from build123d import *

# Parameters (mm, degrees)
SKETCH1_W           = 35
SKETCH1_H           = 18
BOSS_EXTRUDE1_DEPTH = 2
SKETCH2_W           = 5
SKETCH2_H           = 6
BOSS_EXTRUDE2_DEPTH = 1.2
SKETCH3_W           = 5
SKETCH3_H           = 1
BOSS_EXTRUDE3_DEPTH = 1


with BuildPart() as part:
    # Sketch1 → Boss-Extrude1 (new body)
    with BuildSketch(Plane(origin=(0, 0, 0), x_dir=(1, 0, 0), z_dir=(0, 1, 0))):
        Rectangle(SKETCH1_W, SKETCH1_H)
    extrude(amount=BOSS_EXTRUDE1_DEPTH)

    # Sketch2 → Boss-Extrude2 (add)
    with BuildSketch(Plane(origin=(17.5, 0, 0), x_dir=(0, 0, -1), z_dir=(1, 0, 0))):
        with Locations((0, -3)):
            Rectangle(SKETCH2_W, SKETCH2_H)
    boss_extrude2 = extrude(amount=-BOSS_EXTRUDE2_DEPTH)

    # Sketch3 → Boss-Extrude3 (add)
    with BuildSketch(Plane.ZY.offset(-16.3)):
        with Locations((0, -5.5)):
            Rectangle(SKETCH3_W, SKETCH3_H)
    boss_extrude3 = extrude(amount=BOSS_EXTRUDE3_DEPTH)

    # Mirror1: Boss-Extrude2, Boss-Extrude3 across plane
    add(boss_extrude2.mirror(Plane(origin=(0, 0, 0), x_dir=(0, 0, 1), z_dir=(1, 0, 0))))
    add(boss_extrude3.mirror(Plane(origin=(0, 0, 0), x_dir=(0, 0, 1), z_dir=(1, 0, 0))))


solid = part.part
Check sheet for the modelled part. Datum: model origin and axes. Units: mm. A direction names the side the tool comes from. Give positions to 0.01 mm unless a question says otherwise; leave off trailing zeros. Loops run counter-clockwise (first coordinate to the right, second up) from the corner with the lowest first, then second, coordinate; pieces in that order, holes last. Notation, with made-up numbers: M -40,71 L -2,71 A36 ccw -2,105 Z; hole C 24,69 d6. An arc over 180 degrees is marked long. Use a Markdown table: item, result. Add a question column.
Q1. Sectioned sample at B-B, the plane z = -0.25. Record the cut outline in (x, y), then the cut area to 3 significant figures.
Q2. Sectioned sample at D-D, the plane z = 7.25. Record the cut outline in (x, y).
Q3. Go/stop test with flat-tipped pins: pin 1 (1 mm diameter, centred on x = 1, y = -1, fed in from -Z); pin 2 (1.1 mm diameter, centred on x = 17, y = -2, fed in from +Z); pin 3 (9 mm diameter, centred on x = 5.5, z = -3.5, fed in from -Y); pin 4 (1.8 mm diameter, centred on x = -16, y = -4.5, fed in from -Z). Record where each tip stops, or that it passes through.
Q4. Mould release check, pull along X, two halves, no side actions. Record for faces 5 (the flat face through (16.3, -2, 0)), 6 (the flat face through (16, -6, 0)), 7 (the flat face through (17.5, -1, 0)): pulls with the +X half, pulls with the -X half, needs draft (parallel to the pull), parting line crosses it, or undercut.
Q5. Tool access check on faces 1 (the flat face through (-17, -4, 2.5)), 2 (the flat face through (-15.3, -5.5, 0)), 3 (the flat face through (-17, -4, -2.5)), 4 (the flat face through (16, -5, 0)). Record the directions out of +Z, -Z, +X, -X, +Y, -Y that give a thin tool (end or side, any length) a straight path to the whole face; none if there is none.
Q6. Sectioned sample at A-A, the plane y = -0.5. Record the cut outline in (x, z).
Q7. Sectioned sample at C-C, the plane x = 5. Record the cut outline in (y, z).
Q8. Scan lines: line 1 along X through (y, z) = (-4.5, 0.5); line 2 along Y through (x, z) = (2.5, 4.25). Record each from-to range of solid material in increasing order. Write a range as [from, to].
Verdict:
| question | item | result |
|---|---|---|
| 1 | outline | M -17.5,-6 L -15.3,-6 L -15.3,-5 L -16.3,-5 L -16.3,0 L 16.3,0 L 16.3,-5 L 15.3,-5 L 15.3,-6 L 17.5,-6 L 17.5,2 L -17.5,2 Z |
| 1 | area | 86.4 mm^2 |
| 2 | outline | M -17.5,0 L 17.5,0 L 17.5,2 L -17.5,2 Z |
| 3 | pin 1 | through |
| 3 | pin 2 | z = 2.5 |
| 3 | pin 3 | y = 0 |
| 3 | pin 4 | z = -2.5 |
| 4 | face 5 | undercut |
| 4 | face 6 | needs draft |
| 4 | face 7 | pulls with the +X half |
| 5 | face 1 | +Z, +X, -X, -Y |
| 5 | face 2 | +Z, -Z, -Y |
| 5 | face 3 | -Z, +X, -X, -Y |
| 5 | face 4 | +Z, -Z |
| 6 | outline | M -17.5,-2.5 L -16.3,-2.5 L -16.3,2.5 L -17.5,2.5 Z; M 16.3,-2.5 L 17.5,-2.5 L 17.5,2.5 L 16.3,2.5 Z |
| 7 | outline | M 0,-9 L 2,-9 L 2,9 L 0,9 Z |
| 8 | line 1 | [-17.5, -16.3], [16.3, 17.5] |
| 8 | line 2 | [0, 2] |
